```python
from build123d import *

# Parameters (mm, degrees)
CASE_SKETCH_W      = 40
CASE_SKETCH_H      = 39.9
CASE_2_DEPTH       = 20
TABS_SKETCH_W      = 8.25
TABS_SKETCH_H      = 2.5
TABS_DEPTH         = 20
SHAFT_SKETCH_W     = 3
SHAFT_SKETCH_H     = 4
TAB_HOLES_SKETCH_R = 1.6
TAB_HOLES_DEPTH    = 53.1


with BuildPart() as part:
    # Case Sketch → Case 2 (new body)
    with BuildSketch(Plane.XY.offset(14)):
        with Locations((-10, 37.55)):
            Rectangle(CASE_SKETCH_W, CASE_SKETCH_H)
    extrude(amount=CASE_2_DEPTH)

    # Tabs Sketch → Tabs (add)
    with BuildSketch(Plane.XY.offset(14)):
        with Locations((-34.125, 46.85)):
            Rectangle(TABS_SKETCH_W, TABS_SKETCH_H)
        with Locations((14.125, 46.85)):
            Rectangle(TABS_SKETCH_W, TABS_SKETCH_H)
    extrude(amount=TABS_DEPTH)

    # Shaft Sketch → Shaft (revolve)
    with BuildSketch(Plane.XY.offset(24), mode=Mode.PRIVATE) as shaft_sk:
        with Locations((1.5, 59.5)):
            Rectangle(SHAFT_SKETCH_W, SHAFT_SKETCH_H)
    revolve(shaft_sk.sketch.rotate(Axis((0, -100, 24), (0, 1, 0)), 90), axis=Axis((0, -100, 24), (0, 1, 0)))

    # Tab Holes Sketch → Tab Holes (cut, symmetric)
    with BuildSketch(Plane(origin=(0, 0, 0), x_dir=(1, 0, 0), z_dir=(0, 1, 0))):
        with Locations(Location((-34.75, -19, 0), (0, 0, 270))):
            Circle(TAB_HOLES_SKETCH_R)
        with Locations(Location((-34.75, -29, 0), (0, 0, 270))):
            Circle(TAB_HOLES_SKETCH_R)
        with Locations(Location((14.75, -19, 0), (0, 0, 270))):
            Circle(TAB_HOLES_SKETCH_R)
        with Locations(Location((14.75, -29, 0), (0, 0, 270))):
            Circle(TAB_HOLES_SKETCH_R)
    extrude(amount=TAB_HOLES_DEPTH, both=True, mode=Mode.SUBTRACT)


solid = part.part
```
Geometry: final body of the model. Coordinates: model frame, mm. A direction names the side the tool comes from. Give positions to 0.01 mm unless a question says otherwise; leave off trailing zeros. Write each loop counter-clockwise with the first axis right and the second up, starting at its lowest first coordinate (ties: lowest second). Pieces come first, ordered by that corner, then holes.
1. Draft query along X for faces 5 (the cylindrical face through (-36, 47, 28)), 6 (the flat face through (-10, 38, 34)), 7 (the flat face through (-38.25, 47, 24)). Return one class per face: released by +X, released by -X, zero draft, split by the parting line, or undercut.
2. Section query A-A, the plane z = 19. Return loops of the section in (x, y).
3. Reachability of faces 1 (the flat face through (-34, 48.1, 24)), 2 (the flat face through (10, 31, 24)), 3 (the flat face through (10, 53, 24)), 4 (the flat face through (-34, 45.6, 24)) from +Z, -Z, +X, -X, +Y, -Y: full face, straight path, thin tool, end or side. Return the list, or none.
4. Line query: probe 1 along X at (y, z) = (46.65, 29); probe 2 along Z at (x, y) = (-34.75, 47.2); probe 3 along Z at (x, y) = (14, 47.5). Output: solid intervals per line, ascending.
5. Section query D-D, the plane z = 28.25. Return loops of the section in (x, y), then the cut area to 3 significant figures.
6. Section query B-B, the plane x = 14.75. Return loops of the section in (y, z).
7. Section query C-C, the plane z = 24. Return loops of the section in (x, y), then the cut area to 3 significant figures.
8. Pin query (flat end, axial travel): P1, Ø1.9, axis at x = 14.75, z = 29, coming from the +Y side; P2, Ø6, axis at y = 52, z = 25.5, coming from the +X side; P3, Ø4, axis at x = 13.5, z = 26.5, coming from the -Y side; P4, Ø4, axis at y = 54.5, z = 22, coming from the -X side. Return the tip coordinate at first contact, or that it passes through.
Computed:
1. face 5: undercut
1. face 6: zero draft
1. face 7: released by -X
2. outline: (-38.25, 45.6) - (-36.35, 45.6) - (-36.35, 48.1) - (-38.25, 48.1) - close; (-33.15, 45.6) - (-30, 45.6) - (-30, 17.6) - (10, 17.6) - (10, 45.6) - (13.15, 45.6) - (13.15, 48.1) - (10, 48.1) - (10, 57.5) - (-30, 57.5) - (-30, 48.1) - (-33.15, 48.1) - close; (16.35, 45.6) - (18.25, 45.6) - (18.25, 48.1) - (16.35, 48.1) - close
3. face 1: +Z, -Z, -X, +Y
3. face 2: +Z, -Z, +X, -Y
3. face 3: +Z, -Z, +X, +Y
3. face 4: +Z, -Z, -X, -Y
4. probe 1: x = -38.25 to -36.35, -33.15 to 13.15, 16.35 to 18.25
4. probe 2: z = 14 to 17.4, 20.6 to 27.4, 30.6 to 34
4. probe 3: z = 14 to 17.59, 20.41 to 27.59, 30.41 to 34
5. outline: (-38.25, 45.6) - (-36.16, 45.6) - (-36.16, 48.1) - (-38.25, 48.1) - close; (-33.34, 45.6) - (-30, 45.6) - (-30, 17.6) - (10, 17.6) - (10, 45.6) - (13.34, 45.6) - (13.34, 48.1) - (10, 48.1) - (10, 57.5) - (-30, 57.5) - (-30, 48.1) - (-33.34, 48.1) - close; (16.16, 45.6) - (18.25, 45.6) - (18.25, 48.1) - (16.16, 48.1) - close
5. area: 1,620 mm2
6. outline: (45.6, 14) - (48.1, 14) - (48.1, 17.4) - (45.6, 17.4) - close; (45.6, 20.6) - (48.1, 20.6) - (48.1, 27.4) - (45.6, 27.4) - close; (45.6, 30.6) - (48.1, 30.6) - (48.1, 34) - (45.6, 34) - close
7. outline: (-38.25, 45.6) - (-30, 45.6) - (-30, 17.6) - (10, 17.6) - (10, 45.6) - (18.25, 45.6) - (18.25, 48.1) - (10, 48.1) - (10, 57.5) - (3, 57.5) - (3, 61.5) - (-3, 61.5) - (-3, 57.5) - (-30, 57.5) - (-30, 48.1) - (-38.25, 48.1) - close
7. area: 1,660 mm2
8. P1: passes through
8. P2: stops at x = 10
8. P3: stops at y = 45.6
8. P4: stops at x = -30
